```python
from build123d import *

# Parameters (mm, degrees)
SKETCH1_R           = 70
SKETCH1_R_2         = 50
SKETCH1_R_3         = 10
BOSS_EXTRUDE1_DEPTH = 20
SKETCH1_3_R         = 50
SKETCH1_3_R_2       = 10
BOSS_EXTRUDE2_DEPTH = 70
SKETCH2_R           = 3
CUT_EXTRUDE1_DEPTH  = 71


with BuildPart() as part:
    # Sketch1 → Boss-Extrude1 (new body)
    with BuildSketch(Plane(origin=(0, 0, 0), x_dir=(1, 0, 0), z_dir=(0, 1, 0))):
        Circle(SKETCH1_R)
        Circle(SKETCH1_R_2, mode=Mode.SUBTRACT)
        Circle(SKETCH1_R_2)
        Circle(SKETCH1_R_3, mode=Mode.SUBTRACT)
    extrude(amount=BOSS_EXTRUDE1_DEPTH)

    # Sketch1_3 → Boss-Extrude2 (add)
    with BuildSketch(Plane(origin=(0, 0, 0), x_dir=(1, 0, 0), z_dir=(0, 1, 0))):
        Circle(SKETCH1_3_R)
        Circle(SKETCH1_3_R_2, mode=Mode.SUBTRACT)
    extrude(amount=BOSS_EXTRUDE2_DEPTH)

    # Sketch2 → Cut-Extrude1 (cut, through all)
    with BuildSketch(Plane.XZ):
        with Locations((0, 62.5)):
            Circle(SKETCH2_R)
        with Locations((44.194173824, 44.194173824)):
            Circle(SKETCH2_R)
        with Locations((62.5, 0)):
            Circle(SKETCH2_R)
        with Locations((44.194173824, -44.194173824)):
            Circle(SKETCH2_R)
        with Locations((0, -62.5)):
            Circle(SKETCH2_R)
        with Locations((-44.194173824, -44.194173824)):
            Circle(SKETCH2_R)
        with Locations((-62.5, 0)):
            Circle(SKETCH2_R)
        with Locations((-44.194173824, 44.194173824)):
            Circle(SKETCH2_R)
    extrude(amount=-CUT_EXTRUDE1_DEPTH, mode=Mode.SUBTRACT)


solid = part.part
```
Check sheet for the modelled part. Datum: model origin and axes. Units: mm. A direction names the side the tool comes from. Round coordinates to 2 decimals unless told otherwise and drop trailing zeros. Loops run counter-clockwise (first coordinate to the right, second up) from the corner with the lowest first, then second, coordinate; pieces in that order, holes last. Notation, with made-up numbers: (-37.5, 2) - (-9.5, 2) arc R25 ccw to (-9.5, 31) - close; hole circle Ø8 at (67.25, 27.25). An arc over 180 degrees is marked (long way). Answer as a JSON object with one key per item and string values. Group by question number.
Q1. Sectioned sample at B-B, the plane z = 0. Enter the section's corners in (x, y).
Q2. Mould release check, pull along X, two halves, no side actions. Record for faces 3 (the face through (-55.55, 9.86, 42.594)), 4 (the face through (-0.7, 70, 10.4)), 5 (the face through (-2.17, 34.51, 9.76)): released by +X, released by -X, zero draft, split by the parting line, or undercut.
Q3. Sectioned sample at D-D, the plane z = -62.5. Enter the section's corners in (x, y).
Q4. Scan lines: line 1 along Z through (x, y) = (0, 44); line 2 along X through (y, z) = (10, 6). Record each from-to range of solid material in increasing order. Write a range as [from, to].
Q5. Sectioned sample at C-C, the plane y = 15.5. Count the separate pieces of the cut face and the enclosed holes in it, plus the area to 3 significant figures.
Q6. Set-up check for faces 1 (the face through (-41.42, 9.86, 43.05)), 2 (the face through (47.69, 44.65, -15.02)): record each of +Z, -Z, +X, -X, +Y, -Y from which the full face is reachable in a straight line by a thin tool's end or side.
Q7. Gauge pin test, flat ends, axial feed: P1, Ø5.5, axis at x = 0, z = 62.5, coming from the +Y side; P2, Ø3, axis at y = 20.5, z = -35, coming from the -X side; P3, Ø8, axis at x = 34.5, y = 38.5, coming from the +Z side; P4, Ø8, axis at x = -44.19, z = -44.19, coming from the +Y side. Record the tip position at first contact, or that the pin passes through.
Q8. Sectioned sample at A-A, the plane x = 0. Enter the section's corners in (y, z).
Solution:
{
 "1": {"outline": "(-70, 0) - (-65.5, 0) - (-65.5, 20) - (-70, 20) - close; (-59.5, 0) - (-10, 0) - (-10, 70) - (-50, 70) - (-50, 20) - (-59.5, 20) - close; (10, 0) - (59.5, 0) - (59.5, 20) - (50, 20) - (50, 70) - (10, 70) - close; (65.5, 0) - (70, 0) - (70, 20) - (65.5, 20) - close"},
 "2": {"face 3": "split by the parting line", "face 4": "zero draft", "face 5": "undercut"},
 "3": {"outline": "(-31.52, 0) - (-3, 0) - (-3, 20) - (-31.52, 20) - close; (3, 0) - (31.52, 0) - (31.52, 20) - (3, 20) - close"},
 "4": {"line 1": "z = [-50, -10], [10, 50]", "line 2": "x = [-69.74, -8], [8, 69.74]"},
 "5": {"separate pieces": "1", "enclosed holes": "9", "area": "14,900 mm²"},
 "6": {"face 1": "+Y, -Y", "face 2": "+Y"},
 "7": {"P1": "passes through", "P2": "stops at x = -61.42", "P3": "stops at z = 39.62", "P4": "stops at y = 20"},
 "8": {"outline": "(0, -70) - (20, -70) - (20, -65.5) - (0, -65.5) - close; (0, -59.5) - (20, -59.5) - (20, -50) - (70, -50) - (70, -10) - (0, -10) - close; (0, 10) - (70, 10) - (70, 50) - (20, 50) - (20, 59.5) - (0, 59.5) - close; (0, 65.5) - (20, 65.5) - (20, 70) - (0, 70) - close"}
}
